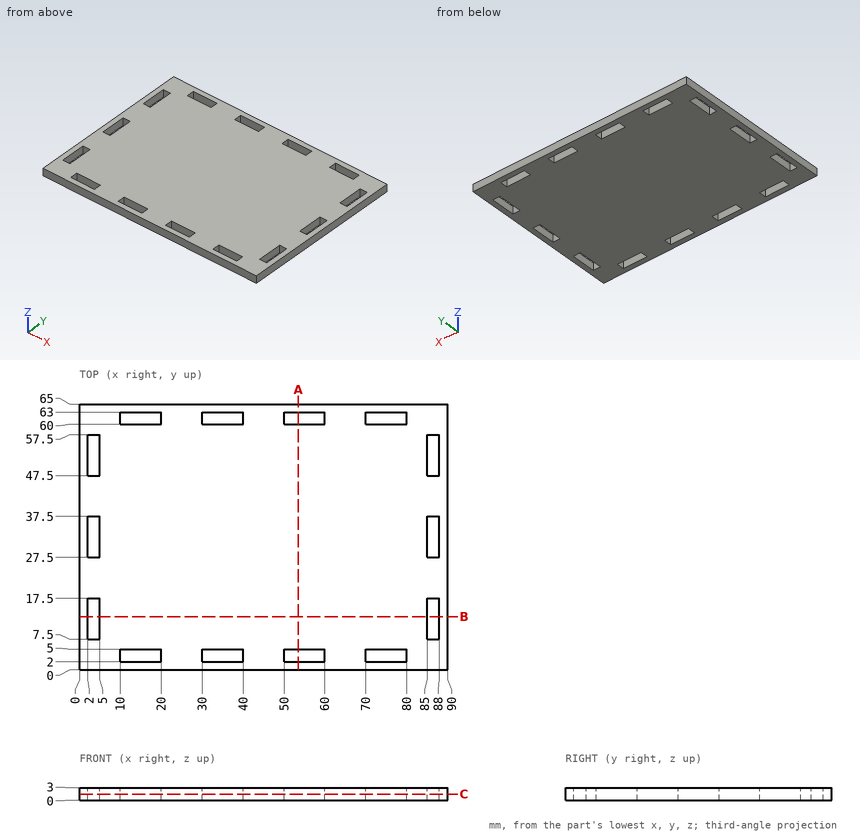
Geometry: see drawing. Coordinates: mm, zero at the bounding-box minimum. Give positions to 0.01 mm unless a question says otherwise; leave off trailing zeros. Order: outer loops, then holes, each group sorted by start corner. A loop starts at its lowest first (then second) coordinate and runs counter-clockwise, first axis right, second up. Notation, with made-up numbers: (-26, 85.25) -> (-4, 85.25) arc R21 cw to (-4, 105.25) -> close; hole circle Ø6 at (28.5, 0.5). An arc over 180 degrees is marked (long way). Write item = value, one per line.
Q1. Cut plane B-B, the plane y = 13. Output: boundary loops of the cut face in (x, z), and give its area (3 significant figures).
Data:
outline = (0, 0) -> (2, 0) -> (2, 3) -> (0, 3) -> close; (5, 0) -> (85, 0) -> (85, 3) -> (5, 3) -> close; (88, 0) -> (90, 0) -> (90, 3) -> (88, 3) -> close
area = 252 mm^2
Q2. Cut plane A-A, the plane x = 53.5. Output: boundary loops of the cut face in (y, z).
Data:
outline = (0, 0) -> (2, 0) -> (2, 3) -> (0, 3) -> close; (5, 0) -> (60, 0) -> (60, 3) -> (5, 3) -> close; (63, 0) -> (65, 0) -> (65, 3) -> (63, 3) -> close
Q3. Material intervals for line 1 (Y direction, x = 77, z = 1.3); line 2 (X direction, y = 29.5, z = 1.4), sorted ascending. Write a range as from..to.
Data:
line_1 = 0..2, 5..60, 63..65
line_2 = 0..2, 5..85, 88..90
Q4. Cut plane C-C, the plane z = 1.5. State how many separate pieces and enclosed holes the cut face has, and give its area (3 significant figures).
Data:
separate_pieces = 1
enclosed_holes = 14
area = 5,430 mm^2
